The listing builds one solid part. Answer for the finished solid, in the listing's coordinates (mm). A direction names the side the tool comes from. Coordinates: 2 decimals unless noted, no trailing zeros. Order: outer loops, then holes, each group sorted by start corner. A loop starts at its lowest first (then second) coordinate and runs counter-clockwise, first axis right, second up. Notation, with made-up numbers: (10.5, 52.5) - (40.5, 52.5) arc R9 ccw to (40.5, 57.5) - close; hole circle Ø5 at (10.5, 13). An arc over 180 degrees is marked (long way). Use one line per item in the form item = value. Start each with the question number.
Item 1: The mould has two halves that part along X. Classify faces 1 (the cylindrical face through (-0.488, -23.196, 3.549)), 2 (the flat face through (14.7, 15, 3.5)), 3 (the flat face through (-6, -6, 0)): released by +X, released by -X, zero draft, split by the parting line, or undercut.
Item 2: A tool of negligible diameter and unlimited length cuts with its end or side. For faces 4 (the flat face through (0, -26.87, 3)), 5 (the cylindrical face through (2.213, -16.855, 11.056)), from which of +Z, -Z, +X, -X, +Y, -Y can it reach the whole face along a straight path? Write none if from no direction.
Item 3: Section B-B, the plane z = 4 is taken. Write down the section's boundary in (x, y), and give its area (3 significant figures).
Item 4: Section A-A, the plane x = 0 is taken. Write down the section's boundary in (y, z).
Item 5: Consider line 1 along Y through (x, z) = (0, 1.75); line 2 along Z through (x, y) = (-23.5, -3); line 3 along X through (y, z) = (2.5, 11.5). Determine where each line is inside the solid, lowest interval first. Write a range as [from, to].
Item 6: Each of these flat-tipped pins is pushed along its axis until it touches: pin 1 Ø1.5 at (y, z) = (-12.5, 6.5) entering from -X; pin 2 Ø6 at (y, z) = (-14, 12.5) entering from -X; pin 3 Ø3.5 at (x, y) = (0, -21) entering from +Z; pin 4 Ø3 at (y, z) = (-12.5, 4) entering from +X. Where does it stop, or does it pass through?
Item 7: Section D-D, the plane x = -21 is taken. Write down the section's boundary in (y, z).
from build123d import *

# Parameters (mm, degrees)
EXTRUSION1_DEPTH = 7
SKETCH2_R        = 2.25
EXTRUSION2_DEPTH = 20
SKETCH3_R        = 6
EXTRUSION3_DEPTH = 20
EXTRUSION4_START = 8
SKETCH4_R        = 17
SKETCH4_R_2      = 6
EXTRUSION4_DEPTH = 8
CHAMFER1_SIZE    = 4
CHAMFER2_SIZE    = 4
CHAMFER3_SIZE    = 4
CHAMFER4_SIZE    = 4


with BuildPart() as part:
    # Sketch1 → Extrusion1 (new body)
    with BuildSketch(Plane.XY):
        Polygon((-29.69848481, 0), (0, 29.69848481), (29.69848481, 0), (0, -29.69848481), align=None)
    extrude(amount=EXTRUSION1_DEPTH)

    # Sketch2 → Extrusion2 (cut)
    with BuildSketch(Plane.XY.offset(7)):
        with Locations((0, 21)):
            Circle(SKETCH2_R)
        with Locations((21, 0)):
            Circle(SKETCH2_R)
        with Locations((0, -21)):
            Circle(SKETCH2_R)
        with Locations((-21, 0)):
            Circle(SKETCH2_R)
    extrude(amount=-EXTRUSION2_DEPTH, mode=Mode.SUBTRACT)

    # Sketch3 → Extrusion3 (cut)
    with BuildSketch(Plane.XY.offset(7)):
        Circle(SKETCH3_R)
    extrude(amount=-EXTRUSION3_DEPTH, mode=Mode.SUBTRACT)

    # Sketch4 → Extrusion4 (add)
    with BuildSketch(Plane.XY.offset(7).offset(EXTRUSION4_START)):
        with Locations(Location((0, 0, 0), (0, 0, 180))):
            Circle(SKETCH4_R)
        Circle(SKETCH4_R_2, mode=Mode.SUBTRACT)
    extrude(amount=-EXTRUSION4_DEPTH)

    # Chamfer1
    chamfer1_edges = [part.edges().sort_by_distance(p)[0] for p in [
        (0, 29.69848481, 3.5),
    ]]
    chamfer(chamfer1_edges, length=CHAMFER1_SIZE)

    # Chamfer2
    chamfer2_edges = [part.edges().sort_by_distance(p)[0] for p in [
        (29.69848481, 0, 3.5),
    ]]
    chamfer(chamfer2_edges, length=CHAMFER2_SIZE)

    # Chamfer3
    chamfer3_edges = [part.edges().sort_by_distance(p)[0] for p in [
        (-29.69848481, 0, 3.5),
    ]]
    chamfer(chamfer3_edges, length=CHAMFER3_SIZE)

    # Chamfer4
    chamfer4_edges = [part.edges().sort_by_distance(p)[0] for p in [
        (0, -29.69848481, 3.5),
    ]]
    chamfer(chamfer4_edges, length=CHAMFER4_SIZE)


solid = part.part
Response:
q1.face_1 = undercut
q1.face_2 = released by +X
q1.face_3 = zero draft
q2.face_4 = +Z, -Z, +X, -X, -Y
q2.face_5 = +Z
q3.outline = (-26.87, -2.83) - (-2.83, -26.87) - (2.83, -26.87) - (26.87, -2.83) - (26.87, 2.83) - (2.83, 26.87) - (-2.83, 26.87) - (-26.87, 2.83) - close; hole circle Ø4.5 at (-21, 0); hole circle Ø12 at (0, 0); hole circle Ø4.5 at (0, -21); hole circle Ø4.5 at (0, 21); hole circle Ø4.5 at (21, 0)
q3.area = 1,560 mm2
q4.outline = (-26.87, 0) - (-23.25, 0) - (-23.25, 7) - (-26.87, 7) - close; (-18.75, 0) - (-6, 0) - (-6, 15) - (-17, 15) - (-17, 7) - (-18.75, 7) - close; (6, 0) - (18.75, 0) - (18.75, 7) - (17, 7) - (17, 15) - (6, 15) - close; (23.25, 0) - (26.87, 0) - (26.87, 7) - (23.25, 7) - close
q5.line_1 = [-26.87, -23.25], [-18.75, -6], [6, 18.75], [23.25, 26.87]
q5.line_2 = [0, 7]
q5.line_3 = [-16.82, -5.45], [5.45, 16.82]
q6.pin_1 = -17.95
q6.pin_2 = -12.96
q6.pin_3 = through
q6.pin_4 = 18.7
q7.outline = (-8.7, 0) - (-2.25, 0) - (-2.25, 7) - (-8.7, 7) - close; (2.25, 0) - (8.7, 0) - (8.7, 7) - (2.25, 7) - close
